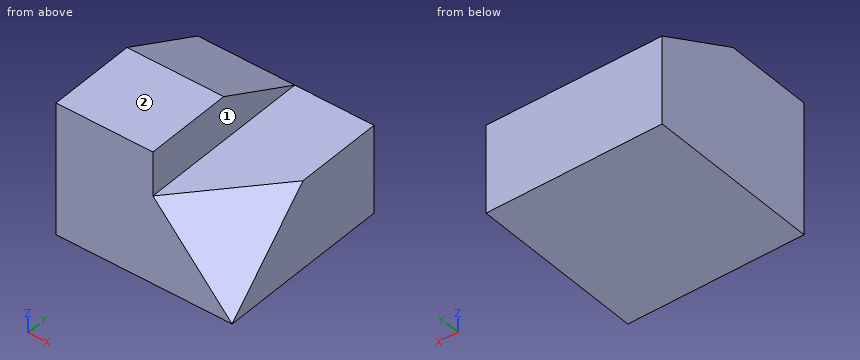
from build123d import *

# Parameters (mm, degrees)
F2_DEPTH  = 127
F3_DEPTH  = 12.7
F0_W      = 139.7
F0_H      = 127
F4_DEPTH  = 31.75
F5_DEPTH  = 95.25
F6_DEPTH  = 31.75
F7_DEPTH  = 95.25
F8_DEPTH  = 31.75
F9_DEPTH  = 95.25
F13_DEPTH = 185.674


with BuildPart() as f2:
    # F1 (on Right) → F2 (new body)
    with BuildSketch(Plane.YZ):
        Polygon((0, 31.75), (127, 31.75), (0, 95.25), (-127, 95.25), (-127, 31.75), align=None)
    extrude(amount=-F2_DEPTH)

    # F1 (on Right) → F3 (join)
    with BuildSketch(Plane.YZ):
        Polygon((0, 31.75), (127, 31.75), (0, 95.25), (-127, 95.25), (-127, 31.75), align=None)
    extrude(amount=F3_DEPTH)

    # F0 (on Top) → F4 (join)
    with BuildSketch(Plane.XY):
        with Locations((-57.15, -63.5)):
            Rectangle(F0_W, F0_H)
        with Locations((-57.15, 63.5)):
            Rectangle(F0_W, F0_H)
    extrude(amount=F4_DEPTH)

    # F0 (on Top) → F5 (join)
    with BuildSketch(Plane.XY):
        with Locations((-57.15, -63.5)):
            Rectangle(F0_W, F0_H)
        with Locations((-57.15, 63.5)):
            Rectangle(F0_W, F0_H)
    extrude(amount=-F5_DEPTH)

    # F0 (on Top) → F6 (join)
    with BuildSketch(Plane.XY):
        Polygon((12.7, 0), (12.7, -127), (127, 0), (127, 127), (12.7, 127), align=None)
    extrude(amount=F6_DEPTH)

    # F0 (on Top) → F7 (join)
    with BuildSketch(Plane.XY):
        Polygon((12.7, 0), (12.7, -127), (127, 0), (127, 127), (12.7, 127), align=None)
    extrude(amount=-F7_DEPTH)

    # F0 (on Top) → F8 (join)
    with BuildSketch(Plane.XY):
        with Locations((-57.15, -63.5)):
            Rectangle(F0_W, F0_H)
        Polygon((127, 0), (12.7, -127), (127, -127), align=None)
        Polygon((12.7, 0), (12.7, -127), (127, 0), (127, 127), (12.7, 127), align=None)
        with Locations((-57.15, 63.5)):
            Rectangle(F0_W, F0_H)
    extrude(amount=F8_DEPTH)

    # F0 (on Top) → F9 (join)
    with BuildSketch(Plane.XY):
        Polygon((127, 0), (12.7, -127), (127, -127), align=None)
    extrude(amount=-F9_DEPTH)

    # F12 (on 3pt) → F13 (cut)
    with BuildSketch(Plane(origin=(59.3797709924, -53.4417938931, 53.4417938931), x_dir=(0.4132877914, 0.8311676694, 0.3719590123), z_dir=(0.6178020632, -0.5560218569, 0.5560218569))):
        Polygon((-88.4998404232, -155.7572883461), (64.2972481493, -61.3589317727), (-88.4998404232, 15.1037370517), align=None)
    extrude(amount=F13_DEPTH, mode=Mode.SUBTRACT)


solid = f2.part
Geometry: final body of the model. Coordinates: model frame, mm. Face numbers are marked on the shaded views. A direction names the side the tool comes from. Give positions to 0.01 mm unless a question says otherwise; leave off trailing zeros. Order: outer loops, then holes, each group sorted by start corner. A loop starts at its lowest first (then second) coordinate and runs counter-clockwise, first axis right, second up. Notation, with made-up numbers: (36, 11) -> (57, 11) arc R25 ccw to (57, 35) -> close; hole circle Ø8 at (-15.75, 85). An arc over 180 degrees is marked (long way). Answer as a JSON object with one key per item and string values.
Q1. Access query for the marked faces 1 and 2. Directions: +Z, -Z, +X, -X, +Y, -Y. A direction counts if a zero-diameter tool reaches every point of the face in a straight line with its end or side. Return the directions, or none.
Entries:
{"face 1": "+Z, +X, +Y, -Y", "face 2": "+Z, +X, -X, +Y, -Y"}
Q2. Section B-B (x = -19). Output: boundary loops of the cut face in (y, z).
Entries:
{"outline": "(-127, -95.25) -> (127, -95.25) -> (127, 31.75) -> (0, 95.25) -> (-127, 95.25) -> close"}
Q3. First-contact query: pin 1 (10 mm diameter, centred on x = 62, z = -15, fed in from -Y); pin 2 (6 mm diameter, centred on y = -28, z = 59, fed in from +X); pin 3 (2 mm diameter, centred on x = 18.5, y = -32.5, fed in from +Z). Flat tips, straight axial feed; report the tip coordinate or a pass-through.
Entries:
{"pin 1": "stops at y = -126.45", "pin 2": "stops at x = 12.7", "pin 3": "stops at z = 31.75"}
Q4. Material intervals for probe 1 along Z at (x, y) = (67, -50); probe 2 along X at (y, z) = (-38.5, 85.5), sorted ascending.
Entries:
{"probe 1": "z = -95.25 to 31.75", "probe 2": "x = -127 to 12.7"}
Q5. Section C-C (z = 60). Output: boundary loops of the cut face in (x, y), plus the area to 3 significant figures.
Entries:
{"outline": "(-127, -127) -> (12.7, -127) -> (12.7, 70.5) -> (-127, 70.5) -> close", "area": "27,600 mm^2"}
Q6. Section D-D (y = -91.5). Output: boundary loops of the cut face in (x, z), plus the area to 3 significant figures.
Entries:
{"outline": "(-127, -95.25) -> (127, -95.25) -> (127, -59.75) -> (44.65, 31.75) -> (12.7, 31.75) -> (12.7, 95.25) -> (-127, 95.25) -> close", "area": "37,400 mm^2"}
Q7. Section A-A (y = -21). Output: boundary loops of the cut face in (x, z).
Entries:
{"outline": "(-127, -95.25) -> (127, -95.25) -> (127, 10.75) -> (108.1, 31.75) -> (12.7, 31.75) -> (12.7, 95.25) -> (-127, 95.25) -> close"}
